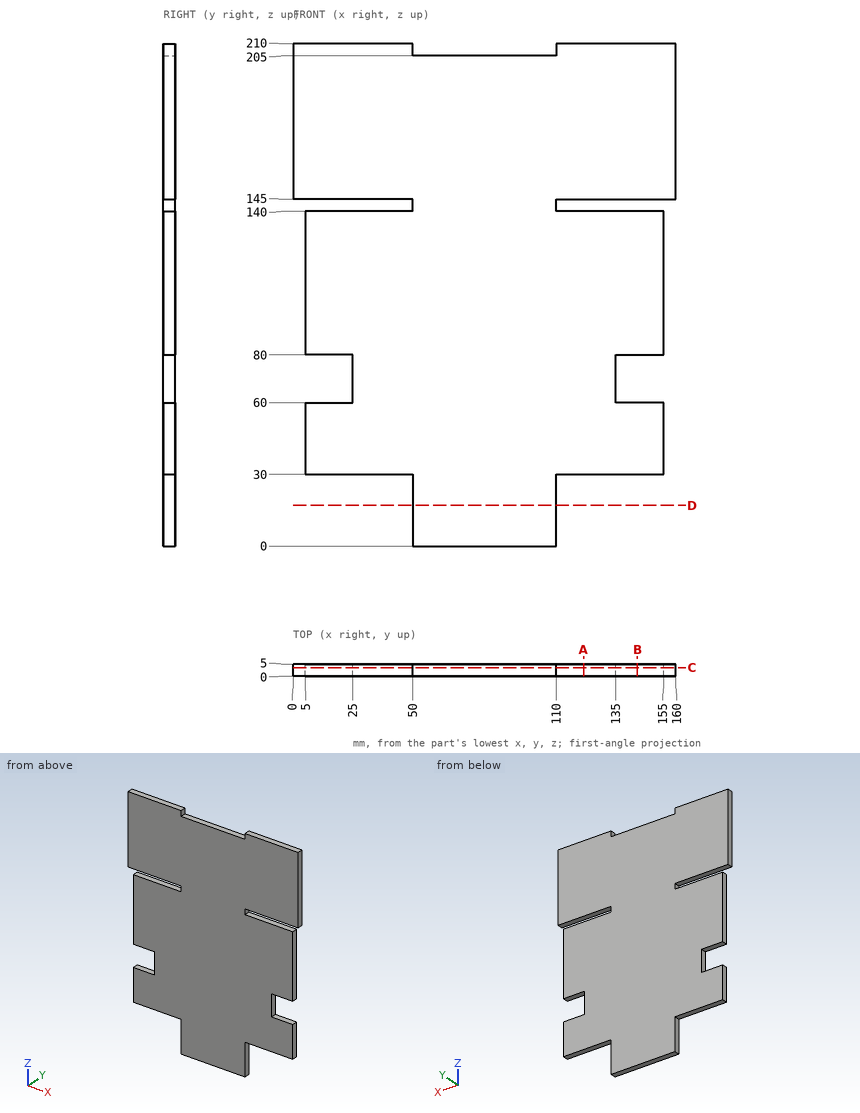
Geometry: see drawing. Coordinates: mm, zero at the bounding-box minimum. Round coordinates to 2 decimals unless told otherwise and drop trailing zeros. Write each loop counter-clockwise with the first axis right and the second up, starting at its lowest first coordinate (ties: lowest second). Pieces come first, ordered by that corner, then holes.
Item 1: Section query C-C (y = 3.5). Return loops of the section in (x, z).
Item 2: Section query B-B (x = 144). Return loops of the section in (y, z).
Item 3: Pin query (flat end, axial travel): P1, Ø1.5, axis at x = 21, y = 2, coming from the -Z side; P2, Ø1.5, axis at y = 2, z = 105, coming from the +X side; P3, Ø2.5, axis at y = 3, z = 71, coming from the -X side. Return the tip coordinate at first contact, or that it passes through.
Item 4: Material intervals for L1, parallel to Z at x = 148, y = 4.1; L2, parallel to Z at x = 128, y = 2.5; L3, parallel to X at y = 1.3, z = 80.5, sorted ascending.
Item 5: Section query D-D (z = 17). Return loops of the section in (x, y), plus the area to 3 significant figures.
Item 6: Section query A-A (x = 121.5). Return loops of the section in (y, z), plus the area to 3 significant figures.
Completed:
1. outline: (0, 145) - (50, 145) - (50, 140) - (5, 140) - (5, 80) - (25, 80) - (25, 60) - (5, 60) - (5, 30) - (50, 30) - (50, 0) - (110, 0) - (110, 30) - (155, 30) - (155, 60) - (135, 60) - (135, 80) - (155, 80) - (155, 140) - (110, 140) - (110, 145) - (160, 145) - (160, 210) - (110, 210) - (110, 205) - (50, 205) - (50, 210) - (0, 210) - close
2. outline: (0, 30) - (5, 30) - (5, 60) - (0, 60) - close; (0, 80) - (5, 80) - (5, 140) - (0, 140) - close; (0, 145) - (5, 145) - (5, 210) - (0, 210) - close
3. P1: stops at z = 30
3. P2: stops at x = 155
3. P3: stops at x = 25
4. L1: z = 30 to 60, 80 to 140, 145 to 210
4. L2: z = 30 to 140, 145 to 210
4. L3: x = 5 to 155
5. outline: (50, 0) - (110, 0) - (110, 5) - (50, 5) - close
5. area: 300 mm2
6. outline: (0, 30) - (5, 30) - (5, 140) - (0, 140) - close; (0, 145) - (5, 145) - (5, 210) - (0, 210) - close
6. area: 875 mm2
